Geometry check sheet. Reference: the model listing, model coordinates, mm. Coordinates: 2 decimals unless noted, no trailing zeros. Write each loop counter-clockwise with the first axis right and the second up, starting at its lowest first coordinate (ties: lowest second). Pieces come first, ordered by that corner, then holes. Notation, with made-up numbers: M 25.25,-17 L 33.25,-17 A6 ccw 33.25,-9 Z; hole C -31,46.5 d7. An arc over 180 degrees is marked long. Answer as a JSON object with one key per item and string values. Group by question number.
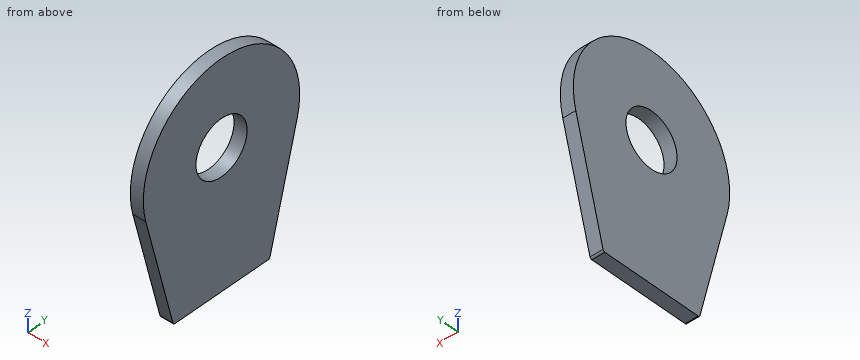
```python
from build123d import *

# Parameters (mm, degrees)
SKETCH1_R             = 6.749999962
BOSS_EXTRUDE1_DEPTH   = 1.5875
FILLET1_R             = 0.508
FILLET2_R             = 0.508
M12_CLEARANCE_HOLE1_D = 13.5


with BuildPart() as part:
    # Sketch1 → Boss-Extrude1 (new, symmetric)
    # profile 1 of 2: a face of its own
    with BuildSketch(Plane(origin=(0, 0, 0), x_dir=(0, 0, -1), z_dir=(1, 0, 0))):
        with BuildLine():
            Line((33.3375, -12.7), (5.163771309, -19.981037814))
            ThreePointArc((5.163771309, -19.981037814), (-20.6375, 0), (5.163771309, 19.981037814))
            Line((5.163771309, 19.981037814), (33.3375, 12.7))
            Line((33.3375, 12.7), (33.3375, -12.7))
        make_face()
        Circle(SKETCH1_R, mode=Mode.SUBTRACT)
    # profile 2 of 2: a face of its own
    with BuildSketch(Plane(origin=(0, 0, 0), x_dir=(0, 0, -1), z_dir=(1, 0, 0))):
        Circle(SKETCH1_R)
    extrude(amount=BOSS_EXTRUDE1_DEPTH, both=True)

    # Fillet1
    fillet1_edges = [part.edges().sort_by_distance(p)[0] for p in [
        (0, -12.7, -33.3375),
    ]]
    fillet(fillet1_edges, radius=FILLET1_R)

    # Fillet2
    fillet2_edges = [part.edges().sort_by_distance(p)[0] for p in [
        (0, 12.7, -33.3375),
    ]]
    fillet(fillet2_edges, radius=FILLET2_R)

    # M12 Clearance Hole1 (through all)
    with Locations(Plane.ZY.offset(1.5875)):
        with Locations((0, 0)):
            Hole(M12_CLEARANCE_HOLE1_D / 2)


solid = part.part
```
1) Section check A-A (z = 0). Record the cut outline in (x, y).
2) Material ranges on probe 1 along Y at (x, z) = (0.3, 0); probe 2 along Y at (x, z) = (1.4, -2); probe 3 along Z at (x, y) = (0.4, 4.5), recorded low to high. Write a range as [from, to].
3) Section check D-D (z = -30). Record the cut outline in (x, y).
4) Go/stop test with a flat-tipped pin: pin 1 Ø12 at (y, z) = (0, 0) entering from -X. Record where the tip stops, or that it passes through.
5) Section check B-B (y = 0). Record the cut outline in (x, z).
Entries:
{
 "1": {"outline": "M -1.59,-20.64 L 1.59,-20.64 L 1.59,-6.75 L -1.59,-6.75 Z; M -1.59,6.75 L 1.59,6.75 L 1.59,20.64 L -1.59,20.64 Z"},
 "2": {"probe 1": "[-20.64, -6.75], [6.75, 20.64]", "probe 2": "[-20.54, -6.45], [6.45, 20.54]", "probe 3": "[-33.34, -5.03], [5.03, 20.14]"},
 "3": {"outline": "M -1.59,-13.56 L 1.59,-13.56 L 1.59,13.56 L -1.59,13.56 Z"},
 "4": {"pin 1": "through"},
 "5": {"outline": "M -1.59,-33.34 L 1.59,-33.34 L 1.59,-6.75 L -1.59,-6.75 Z; M -1.59,6.75 L 1.59,6.75 L 1.59,20.64 L -1.59,20.64 Z"}
}
